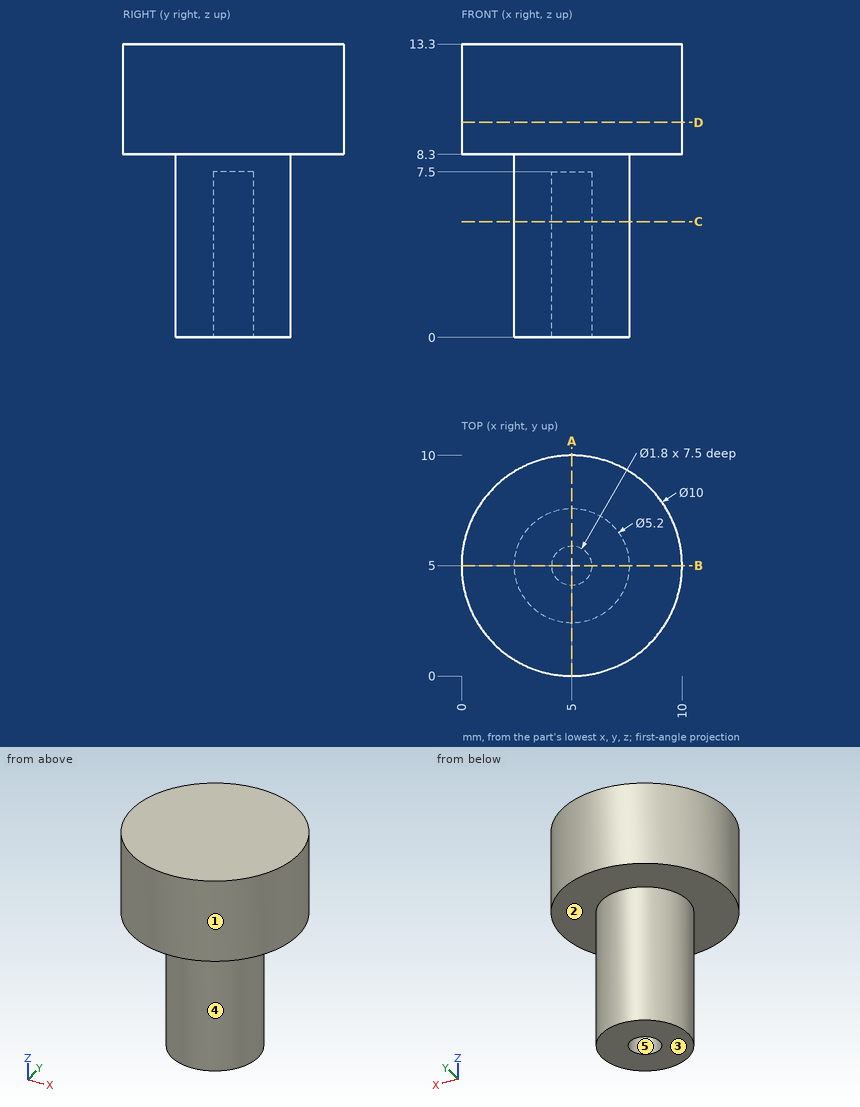
The figure shows three views and two pictorial views of one solid part (mm, origin at its lowest corner). Answer the questions. A direction names the side the tool comes from. Give positions to 0.01 mm unless a question says otherwise; leave off trailing zeros. Write each loop counter-clockwise with the first axis right and the second up, starting at its lowest first coordinate (ties: lowest second). Pieces come first, ordered by that corner, then holes. Notation, with made-up numbers: (-29, 60.25) - (27, 60.25) arc R28 ccw to (27, 86.25) - close; hole circle Ø6 at (34, -30). An arc over 180 degrees is marked (long way). Return JSON: item names as keys, results as strings.
Q1. For a pull along Y with two mould halves and no side action, classify the marked faces 3, 4 and 5 as released by +Y, released by -Y, zero draft, split by the parting line, or undercut.
Reply:
{"face 3": "zero draft", "face 4": "split by the parting line", "face 5": "undercut"}
Q2. A cutting plane is placed at D-D, the plane z = 9.75. Determine the outline of the cut face in (x, y).
Reply:
{"outline": "circle Ø10 at (5, 5)"}
Q3. Given P1, Ø4, axis at x = 8.5, z = 7.5, coming from the +Y side; P2, Ø1, axis at y = 3, z = 7, coming from the -X side; P3, Ø1, axis at y = 7.5, z = 5, coming from the -X side, each flat-ended and moving along its own axis, determine where each tip first touches the part or whether it passes through.
Reply:
{"P1": "y = 9.71", "P2": "x = 2.88", "P3": "x = 3.34"}
Q4. For the marked faces 1 and 2, determine the directions among +Z, -Z, +X, -X, +Y, -Y from which every point of the face is accessible in a straight line to the end or side of a thin tool.
Reply:
{"face 1": "+Z, -Z", "face 2": "-Z"}
Q5. A cutting plane is placed at A-A, the plane x = 5. Determine the outline of the cut face in (y, z), and give its area (3 significant figures).
Reply:
{"outline": "(0, 8.3) - (2.4, 8.3) - (2.4, 0) - (4.1, 0) - (4.1, 7.5) - (5.9, 7.5) - (5.9, 0) - (7.6, 0) - (7.6, 8.3) - (10, 8.3) - (10, 13.3) - (0, 13.3) - close", "area": "79.7 mm²"}
Q6. Consider line 1 along Y through (x, z) = (5, 3.5); line 2 along Z through (x, y) = (8, 8.75); line 3 along X through (y, z) = (5.75, 6.5). Determine where each line is inside the solid, lowest interval first. Write a range as [from, to].
Reply:
{"line 1": "[2.4, 4.1], [5.9, 7.6]", "line 2": "[8.3, 13.3]", "line 3": "[2.51, 4.5], [5.5, 7.49]"}
Q7. A cutting plane is placed at C-C, the plane z = 5.25. Determine the outline of the cut face in (x, y).
Reply:
{"outline": "circle Ø5.2 at (5, 5); hole circle Ø1.8 at (5, 5)"}
